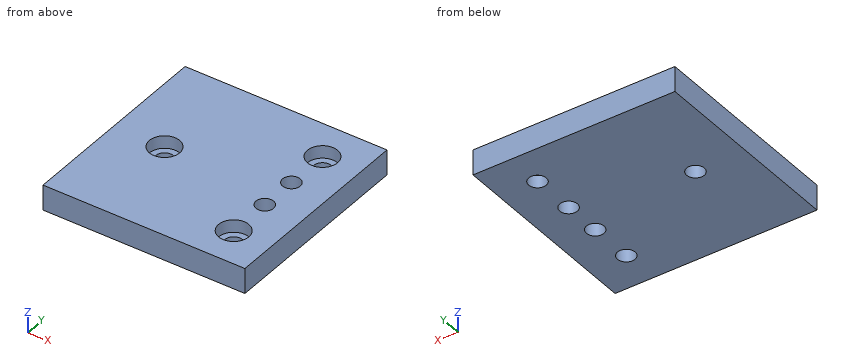
Autodesk Inventor part; units mm, degrees
ref_plane "YZ Plane" through (0, 0, 0) normal (1, 0, 0) x (0, 1, 0)
ref_plane "XZ Plane" through (0, 0, 0) normal (0, 1, 0) x (-1, 0, 0)
ref_plane "XY Plane" through (0, 0, 0) normal (0, 0, 1) x (1, 0, 0)
sketch "Sketch1" plane through (0, 0, 0) normal (0, 0, 1) x (1, 0, 0)
  line L0 (40, -40) -> (-40, -40)
  line L1 (-40, -40) -> (-40, 40)
  line L2 (-40, 40) -> (40, 40)
  line L3 (40, 40) -> (40, -40)
  line L4 (40, -40) -> (-40, 40) construction
  line L5 (-40, -40) -> (40, 40) construction
  point P0 (0, 0)
  dimension "d1" = 80
  dimension "d2" = 80
extrude "Extrusion1" add sketch "Sketch1" along normal mid plane 10
sketch "Sketch2" plane through (0, 0, 5) normal (0, 0, 1) x (1, 0, 0)
  line L0 (-40, 40) -> (-40, -40)
  line L1 (40, 40) -> (-40, 40)
  line L2 (40, -40) -> (40, 40)
  point P0 (0, 0)
  point P1 (25, 25)
  point P2 (25, -25)
  point P3 (-20, 0)
  point P4 (-40, 0)
  dimension "d27" = 15
  dimension "d31" = 15
  dimension "d32" = 50
  dimension "d33" = 40
  dimension "d34" = 20
hole "Hole1" at (25, 25, 5) at (25, -25, 5) at (-20, 0, 5) direction (0, 0, -1) diameter 7 depth 17.1 tip angle 118 counterbore diameter 12 counterbore depth 5
sketch "Sketch3" plane through (0, 0, -5) normal (0, 0, -1) x (-1, 0, 0)
  line L0 (-40, -40) -> (40, -40)
  line L1 (56, 0) -> (-56, 0) construction
  circle A0 centre (-25, 25) radius 3.5
  point P0 (0, 0)
  point P1 (-25, -7.5)
  point P2 (-25, 7.5)
  dimension "d28" = 0
  dimension "d29" = 15
  dimension "d30" = 7.5
hole "Hole2" at (25, -7.5, -5) at (25, 7.5, -5) direction (0, 0, 1) diameter 7 depth 17.1 tip angle 118
properties part number "HCMUTE-CDT23-DE_GA_LOADCELL" material "Stainless Steel"
Check sheet for the modelled part. Datum: model origin and axes. Units: mm. Give positions to 0.01 mm unless a question says otherwise; leave off trailing zeros. Order: outer loops, then holes, each group sorted by start corner. A loop starts at its lowest first (then second) coordinate and runs counter-clockwise, first axis right, second up. Notation, with made-up numbers: M -25,37.25 L 34,37.25 A20 cw 34,59.25 Z; hole C 8,-34.5 d1. An arc over 180 degrees is marked long. Answer in a Markdown table with one row per item.
1) Cross-section at D-D, the plane z = 1.5. Enter the section's corners in (x, y).
Filled sheet:
| item | result |
|---|---|
| outline | M -40,-40 L 40,-40 L 40,40 L -40,40 Z; hole C -20,0 d12; hole C 25,-25 d12; hole C 25,25 d12; hole C 25,-7.5 d7; hole C 25,7.5 d7 |
2) Cross-section at A-A, the plane y = -7.5. Enter the section's corners in (x, z).
Filled sheet:
| item | result |
|---|---|
| outline | M -40,-5 L 21.5,-5 L 21.5,5 L -40,5 Z; M 28.5,-5 L 40,-5 L 40,5 L 28.5,5 Z |
3) Cross-section at B-B, the plane x = 25. Enter the section's corners in (y, z), plus the area to 3 significant figures.
Filled sheet:
| item | result |
|---|---|
| outline | M -40,-5 L -28.5,-5 L -28.5,0 L -31,0 L -31,5 L -40,5 Z; M -21.5,-5 L -11,-5 L -11,5 L -19,5 L -19,0 L -21.5,0 Z; M -4,-5 L 4,-5 L 4,5 L -4,5 Z; M 11,-5 L 21.5,-5 L 21.5,0 L 19,0 L 19,5 L 11,5 Z; M 28.5,-5 L 40,-5 L 40,5 L 31,5 L 31,0 L 28.5,0 Z |
| area | 470 mm2 |
4) Gauge pin test, flat end, axial feed: P1, Ø9, axis at x = 25, y = -25, coming from the +Z side. Record the tip position at first contact, or that the pin passes through.
Filled sheet:
| item | result |
|---|---|
| P1 | stops at z = 0 |
5) Thickness scan on L1, parallel to Y at x = 25, z = -1.8; L2, parallel to Y at x = 25, z = 1.25; L3, parallel to X at y = 0, z = 2.3. Record the ranges inside material, lowest first. Write a range as [from, to].
Filled sheet:
| item | result |
|---|---|
| L1 | y = [-40, -28.5], [-21.5, -11], [-4, 4], [11, 21.5], [28.5, 40] |
| L2 | y = [-40, -31], [-19, -11], [-4, 4], [11, 19], [31, 40] |
| L3 | x = [-40, -26], [-14, 40] |
6) Cross-section at C-C, the plane x = -20. Enter the section's corners in (y, z), plus the area to 3 significant figures.
Filled sheet:
| item | result |
|---|---|
| outline | M -40,-5 L -3.5,-5 L -3.5,0 L -6,0 L -6,5 L -40,5 Z; M 3.5,-5 L 40,-5 L 40,5 L 6,5 L 6,0 L 3.5,0 Z |
| area | 705 mm2 |
